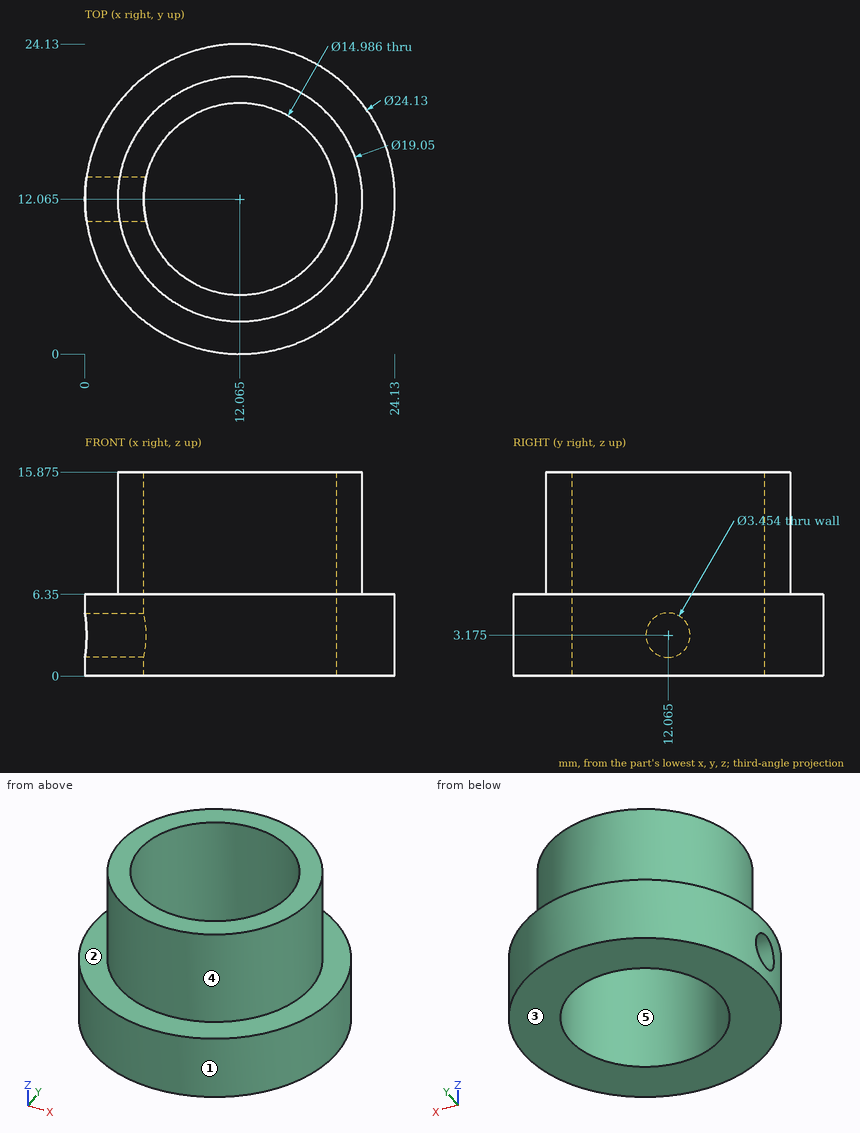
Print and shaded views of the part. All mm, measured from the part's lowest x, y and z. A direction names the side the tool comes from. Round coordinates to 2 decimals unless told otherwise and drop trailing zeros. Use CSV: the item, a comma, the result in double quotes. Start each with the question number.
Item 1: Tool access for the marked faces 1 and 2: list every direction of +Z, -Z, +X, -X, +Y, -Y with a clear straight run to the whole face (end or side of a thin tool).
Item 2: Pin check, flat tips, straight feed: P1, Ø2, axis at x = 3.5, z = 4, coming from the -Y side (1 decimal); P2, Ø2, axis at y = 18, z = 12.5, coming from the +X side; P3, Ø4, axis at x = 9, z = 3.5, coming from the -Y side. Stop position of each tip, or through.
Item 3: Two-plate mould, pull along Y, no slides. Class the marked faces 3, 4 and 5: released by +Y, released by -Y, zero draft, split by the parting line, or undercut.
Item 4: Drill centre lines: L1, parallel to Y at x = 12.25, z = 8 (1 decimal); L2, parallel to Y at x = 17.25, z = 10.5 (1 decimal); L3, parallel to X at y = 15, z = 1.25. Where is each one in solid material? Low to high. Write a range as [from, to].
Checked values:
1,face 1,"+Z, -Z"
1,face 2,"+Z"
2,P1,"stops at y = 2.7"
2,P2,"stops at x = 20.21"
2,P3,"stops at y = 0.05"
3,face 3,"zero draft"
3,face 4,"split by the parting line"
3,face 5,"undercut"
4,L1,"y = [2.5, 4.6], [19.6, 21.6]"
4,L2,"y = [4.1, 6.7], [17.5, 20.1]"
4,L3,"x = [0.36, 5.17], [18.96, 23.77]"
